Source: CAD feature listing. Evaluate the final solid. Frame: model axes, mm. A direction names the side the tool comes from. Round coordinates to 2 decimals unless told otherwise and drop trailing zeros. Put each result on its own line as item: value. Start each with the question number.
```python
from build123d import *

# Parameters (mm, degrees)
F0_W     = 609.6
F0_H     = 609.6
F1_DEPTH = 304.8
F2_R     = 38.1
F3_DEPTH = 25.4


with BuildPart() as f1:
    # F0 (on Front) → F1 (new body, symmetric)
    with BuildSketch(Plane.XZ):
        with Locations((0, -304.8)):
            Rectangle(F0_W, F0_H)
    extrude(amount=F1_DEPTH, both=True)

    # F2 (on face) → F3 (cut)
    with BuildSketch(Plane(origin=(0, 0, -609.6), x_dir=(1, 0, 0), z_dir=(0, 0, -1))):
        Circle(F2_R)
    extrude(amount=-F3_DEPTH, mode=Mode.SUBTRACT)


solid = f1.part
```
(1) Ray query, line 1 along Y through (x, z) = (0, -595.25). Return the intervals inside material, ascending.
(2) Access query for faces 1 (the cylindrical face through (-30.235, 23.183, -597.078)), 2 (the flat face through (304.8, -4, -309)). Directions: +Z, -Z, +X, -X, +Y, -Y. A direction counts if a zero-diameter tool reaches every point of the face in a straight line with its end or side. Return the directions, or none.
(3) Contact query for a flat-ended pin moving along its axis: P1, Ø23, axis at x = 14.5, y = -14.5, coming from the -Z side. Output: stop coordinate, or through.
Entries:
1. line 1: -304.8 to -38.1, 38.1 to 304.8
2. face 1: -Z
2. face 2: +Z, -Z, +X, +Y, -Y
3. P1: z = -584.2
